The figure shows three views and two pictorial views of one solid part (mm, origin at its lowest corner). Answer the questions. A direction names the side the tool comes from. Coordinates: 2 decimals unless noted, no trailing zeros. Loops run counter-clockwise (first coordinate to the right, second up) from the corner with the lowest first, then second, coordinate; pieces in that order, holes last. Notation, with made-up numbers: M -7,74.25 L 39,74.25 A23 cw 39,103.25 Z; hole C 60,29.5 d10. An arc over 180 degrees is marked long. Return JSON: item names as keys, results as strings. Group by question number.
1. Section C-C (y = 58.5) is taken. Write down the section's boundary in (x, z).
2. The mould has two halves that part along Z. Classify the marked faces 1, 2 and 3: pulls with the +Z half, pulls with the -Z half, needs draft (parallel to the pull), parting line crosses it, or undercut.
3. Straight lines are drawn through the part: L1, parallel to X at y = 14, z = 10; L2, parallel to Y at x = 16.25, z = 5; L3, parallel to Y at x = 8.75, z = 6.25. For each, find the intervals that lie inside material, in ascending order. Write a range as from..to.
4. Section A-A (z = 10) is taken. Write down the section's boundary in (x, y), then the cut area to 3 significant figures.
5. Section D-D (z = 6.5) is taken. Write down the section's boundary in (x, y), then the cut area to 3 significant figures.
6. Which of the six approach directions +Z, -Z, +X, -X, +Y, -Y give full straight-line access (tool end or side, diameter ignored) to the marked faces 4 and 5?
7. Given P1, Ø1.5, axis at x = 14.5, y = 77, coming from the -Z side; P2, Ø1.5, axis at y = 39.5, z = 16.5, coming from the +X side; P3, Ø4, axis at y = 34.5, z = 3.5, coming from the +X side; P4, Ø8, axis at x = 10, z = 10, coming from the -Y side, each flat-ended and moving along its own axis, determine where each tip first touches the part or whether it passes through.
8. Section B-B (x = 10) is taken. Write down the section's boundary in (y, z).
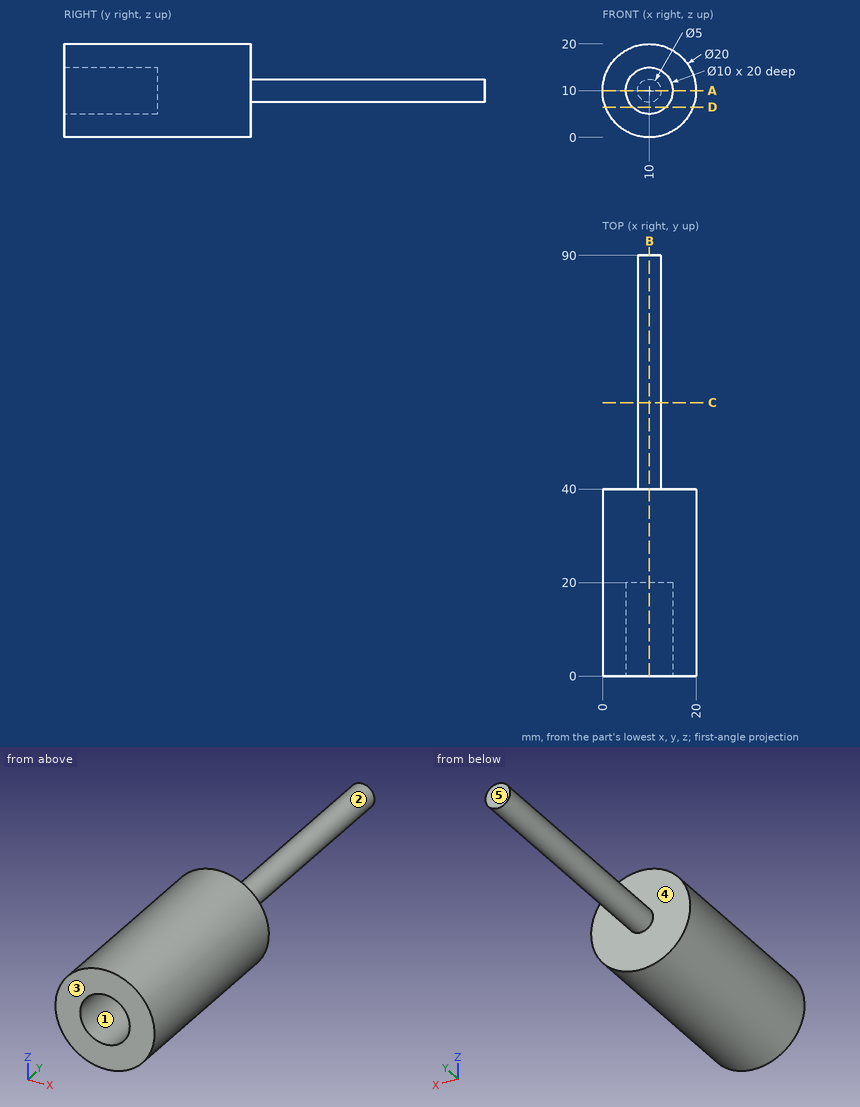
Worked out:
{
 "1": {"outline": "C 10,10 d5"},
 "2": {"face 1": "undercut", "face 2": "parting line crosses it", "face 3": "needs draft"},
 "3": {"L1": "0..5, 15..20", "L2": "0..40", "L3": "20..40"},
 "4": {"outline": "M 0,0 L 5,0 L 5,20 L 15,20 L 15,0 L 20,0 L 20,40 L 12.5,40 L 12.5,90 L 7.5,90 L 7.5,40 L 0,40 Z", "area": "850 mm^2"},
 "5": {"outline": "M 0.63,0 L 6.43,0 L 6.43,20 L 13.57,20 L 13.57,0 L 19.37,0 L 19.37,40 L 0.63,40 Z", "area": "607 mm^2"},
 "6": {"face 4": "+Y", "face 5": "+Z, -Z, +X, -X, +Y"},
 "7": {"P1": "through", "P2": "x = 18.18", "P3": "x = 18.93", "P4": "y = 20"},
 "8": {"outline": "M 0,0 L 40,0 L 40,7.5 L 90,7.5 L 90,12.5 L 40,12.5 L 40,20 L 0,20 L 0,15 L 20,15 L 20,5 L 0,5 Z"}
}
